Can you work these out from the model? Positions are in its coordinate system, mm. Face numbers are marked on the shaded views. A direction names the side the tool comes from. Round coordinates to 2 decimals unless told otherwise and drop trailing zeros. Write each loop counter-clockwise with the first axis right and the second up, starting at its lowest first coordinate (ties: lowest second). Pieces come first, ordered by that corner, then holes. Notation, with made-up numbers: (54, 31) -> (61, 31) arc R6 ccw to (61, 35) -> close; hole circle Ø4 at (-35, 88). An arc over 180 degrees is marked (long way). Use CSV: the item, a comma, the result in double quotes.
```python
from build123d import *

# Parameters (mm, degrees)
F0_R        = 9.525
F1_DEPTH    = 25.4
F3_DEPTH    = 25.4
F1_FACE_R   = 9.525
F1_FACE_R_2 = 4.7625
F4_DEPTH    = 8.8138
F6_DEPTH    = 9.525


with BuildPart() as f1:
    # F0 (on Front) → F1 (new body)
    with BuildSketch(Plane.XZ):
        Circle(F0_R)
    extrude(amount=F1_DEPTH)

    # F2 (on Front) → F3 (cut)
    with BuildSketch(Plane.XZ):
        with BuildLine():
            ThreePointArc((4.7625, 0), (3.3675960454, 3.3675960454), (0, 4.7625))
            ThreePointArc((0, 4.7625), (-3.3675960454, 3.3675960454), (-4.7625, 0))
            ThreePointArc((-4.7625, 0), (-3.3675960454, -3.3675960454), (0, -4.7625))
            ThreePointArc((0, -4.7625), (3.3675960454, -3.3675960454), (4.7625, 0))
        make_face()
    extrude(amount=F3_DEPTH, mode=Mode.SUBTRACT)

    # F2 (on Front) + F1_face (on face) → F4 (cut)
    with BuildSketch(Plane.XZ):
        with BuildLine():
            Line((4.7625, 0), (4.7625, 4.7625))
            Line((4.7625, 4.7625), (0, 4.7625))
            ThreePointArc((0, 4.7625), (3.3675960454, 3.3675960454), (4.7625, 0))
        make_face()
        with BuildLine():
            ThreePointArc((-4.7625, 0), (-3.3675960454, 3.3675960454), (0, 4.7625))
            Line((0, 4.7625), (-4.7625, 4.7625))
            Line((-4.7625, 4.7625), (-4.7625, 0))
        make_face()
        with BuildLine():
            ThreePointArc((4.7625, 0), (3.3675960454, 3.3675960454), (0, 4.7625))
            ThreePointArc((0, 4.7625), (-3.3675960454, 3.3675960454), (-4.7625, 0))
            ThreePointArc((-4.7625, 0), (-3.3675960454, -3.3675960454), (0, -4.7625))
            ThreePointArc((0, -4.7625), (3.3675960454, -3.3675960454), (4.7625, 0))
        make_face()
        with BuildLine():
            Line((4.7625, -4.7625), (4.7625, 0))
            ThreePointArc((4.7625, 0), (3.3675960454, -3.3675960454), (0, -4.7625))
            Line((0, -4.7625), (4.7625, -4.7625))
        make_face()
        with BuildLine():
            ThreePointArc((0, -4.7625), (-3.3675960454, -3.3675960454), (-4.7625, 0))
            Line((-4.7625, 0), (-4.7625, -4.7625))
            Line((-4.7625, -4.7625), (0, -4.7625))
        make_face()
    with BuildSketch(Plane.XZ.offset(25.4)):
        Circle(F1_FACE_R)
        Circle(F1_FACE_R_2, mode=Mode.SUBTRACT)
    extrude(amount=F4_DEPTH, mode=Mode.SUBTRACT)

    # F5 (on face) → F6 (cut)
    with BuildSketch(Plane.XZ.offset(25.4)):
        Polygon((-3.65125, -6.3241505111), (3.65125, -6.3241505111), (7.3025, 0), (3.65125, 6.3241505111), (-3.65125, 6.3241505111), (-7.3025, 0), align=None)
    extrude(amount=-F6_DEPTH, mode=Mode.SUBTRACT)


solid = f1.part
```
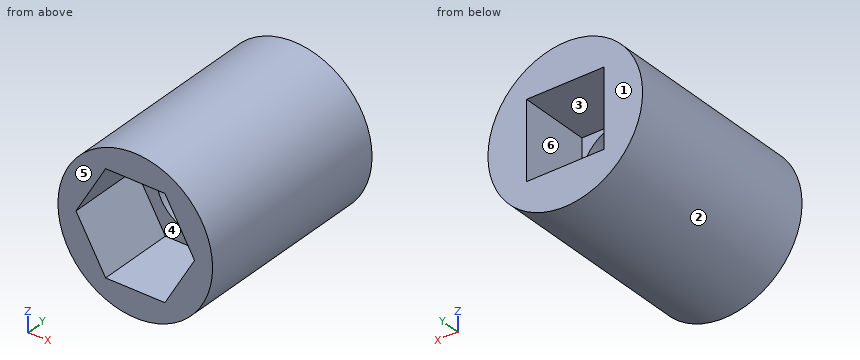
Q1. On a 3-axis mill with a long thin cutter (end or side, diameter ignored), from which of +Z, -Z, +X, -X, +Y, -Y can I reach the whole of each face in a straight line? I mean the marked faces 4, 5 and 6. Say none if no direction works.
Resolved:
face 4,"-Y"
face 5,"+Z, -Z, +X, -X, -Y"
face 6,"+Y"
Q2. Will these pins go through, and if not, where does the flat tip stop? P1, Ø2.5, axis at y = -4.5, z = 1.5, coming from the +X side; P2, Ø10, axis at y = -18.5, z = -7, coming from the +X side; P3, Ø5, axis at y = -12, z = -5, coming from the -X side.
Resolved:
P1,"stops at x = 9.52"
P2,"stops at x = 9.31"
P3,"stops at x = -9.19"
Q3. If we mould it in two halves opening along Z, with no side actions, what happens to the marked faces 1, 2 and 3? For each: released by +Z, released by -Z, zero draft, split by the parting line, or undercut.
Resolved:
face 1,"zero draft"
face 2,"split by the parting line"
face 3,"undercut"
Q4. Suppose I cut it at D-D (x = 6.75). Write out the boundary of the cut face in (y, z) (3 decimals), and give its area (3 significant figures).
Resolved:
outline,"(-25.4, -6.72) -> (0, -6.72) -> (0, 6.72) -> (-25.4, 6.72) -> (-25.4, 0.957) -> (-15.875, 0.957) -> (-15.875, -0.957) -> (-25.4, -0.957) -> close"
area,"323 mm^2"
Q5. Please list where these lines run through material, in increasing order: probe 1 along X at (y, z) = (-11.75, 0.25); probe 2 along Z at (x, y) = (-4, -10.25); probe 3 along X at (y, z) = (-22, -6).
Resolved:
probe 1,"x = -9.52 to -4.76, 4.76 to 9.52"
probe 2,"z = -8.64 to -2.58, 2.58 to 8.64"
probe 3,"x = -7.4 to -3.84, 3.84 to 7.4"
